```python
from build123d import *

# Parameters (mm, degrees)
SKETCH1_R           = 25.4
BOSS_EXTRUDE1_DEPTH = 40.132
BOSS_EXTRUDE1_TAPER = 5
SHELL1_T            = -2.54
SCALE1_SCALE        = 18


with BuildPart() as part:
    # Sketch1 → Boss-Extrude1 (new body)
    with BuildSketch(Plane(origin=(0, 0, 0), x_dir=(0, 0, -1), z_dir=(1, 0, 0))):
        Circle(SKETCH1_R)
    extrude(amount=BOSS_EXTRUDE1_DEPTH, taper=BOSS_EXTRUDE1_TAPER)

    # Shell1
    shell1_openings = [part.faces().sort_by_distance(p)[0] for p in [
        (40.132, 0, 0),
    ]]
    offset(amount=SHELL1_T, openings=shell1_openings, kind=Kind.INTERSECTION)


with BuildPart() as part_1:
    # Scale1: scaled about (15.466911265, 0, 0)
    add(part.part.scale(SCALE1_SCALE).moved(Location((-262.937491505, 0, 0))))


solid = part_1.part
```
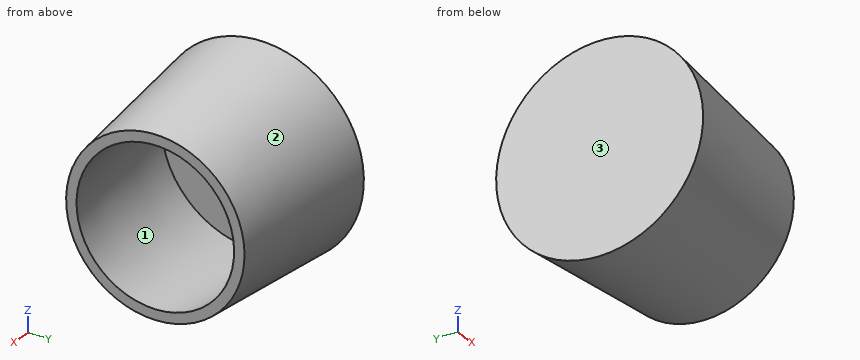
Check sheet for the modelled part. Datum: model origin and axes. Units: mm. Face numbers are marked on the shaded views. Round coordinates to 2 decimals unless told otherwise and drop trailing zeros. Write each loop counter-clockwise with the first axis right and the second up, starting at its lowest first coordinate (ties: lowest second). Pieces come first, ordered by that corner, then holes. Notation, with made-up numbers: (64.5, 64.5) -> (105.5, 64.5) arc R29 cw to (105.5, 87.5) -> close; hole circle Ø7 at (-19.75, -27). An arc over 180 degrees is marked (long way). Put each result on its own line as item: value.
(1) Go/stop test with flat-tipped pins: pin 1 Ø8 at (x, y) = (-176.5, 259) entering from +Z; pin 2 Ø1.5 at (x, y) = (94.5, -296.5) entering from +Z; pin 3 Ø1 at (x, z) = (276, -261.5) entering from +Y. Record where each tip stops, or that it passes through.
Values found:
pin 1: stops at z = 370.37
pin 2: stops at z = 306.51
pin 3: stops at y = 316.26
(2) Sectioned sample at B-B (x = 314). Enter the section's corners in (y, z).
Values found:
outline: circle Ø813.45 at (0, 0); hole circle Ø721.66 at (0, 0)
(3) Sectioned sample at C-C (x = -18.5). Enter the section's corners in (y, z).
Values found:
outline: circle Ø871.63 at (0, 0); hole circle Ø779.84 at (0, 0)
(4) Sectioned sample at A-A (z = 0). Enter the section's corners in (x, y).
Values found:
outline: (-262.94, -457.2) -> (459.44, -394) -> (459.44, -348.11) -> (-217.22, -407.31) -> (-217.22, 407.31) -> (459.44, 348.11) -> (459.44, 394) -> (-262.94, 457.2) -> close
(5) Mould release check, pull along Y, two halves, no side actions. Record for the marked faces 1, 2 and 3: released by +Y, released by -Y, zero draft, split by the parting line, or undercut.
Values found:
face 1: undercut
face 2: split by the parting line
face 3: zero draft
(6) Material ranges on line 1 (X direction, y = -49, z = -144.5); line 2 (Z direction, x = 23, y = -337); line 3 (Z direction, x = -27, y = -254), recorded low to high.
Values found:
line 1: x = -262.94 to -217.22
line 2: z = -270.58 to -188.81, 188.81 to 270.58
line 3: z = -355.06 to -296.82, 296.82 to 355.06
